Work out the finished part from the listing and answer in its coordinate system (mm). Face numbers are marked on the shaded views. A direction names the side the tool comes from. Round coordinates to 2 decimals unless told otherwise and drop trailing zeros.
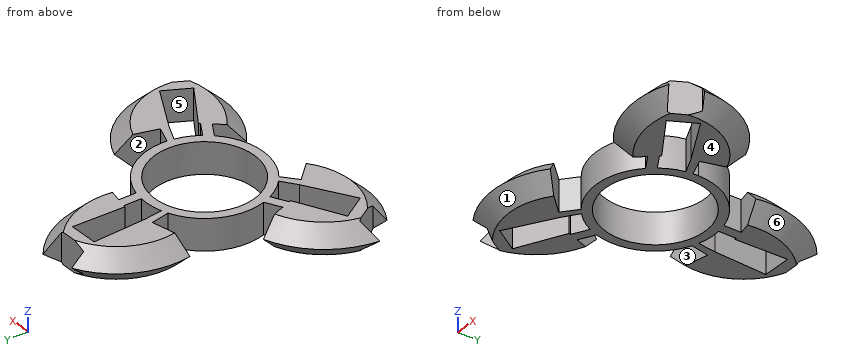
```python
from build123d import *

# Parameters (mm, degrees)
F0_R     = 11.2
F1_DEPTH = 7
F2_SIZE  = 3.5
F3_SIZE  = 3.49999


# Not quite as in the source:
# - a fillet or chamfer is up to 0.001 mm smaller than in the source, because OpenCascade refuses the exact size


with BuildPart() as f1:
    # F0 (on Top) → F1 (new body)
    with BuildSketch(Plane.XY):
        Polygon((-5.4887417888, 30.3404310419), (-5.3626246511, 27.9541106613), (0.7814850479, 28.2788271306), (0.8367048606, 30.6747311771), align=None)
        with BuildLine():
            Line((-6.3603435788, 15.9527909689), (-4.7504720739, 16.3712901342))
            Line((-4.7504720739, 16.3712901342), (-5.3626246511, 27.9541106613))
            Line((-5.3626246511, 27.9541106613), (-5.4887417888, 30.3404310419))
            Line((-5.4887417888, 30.3404310419), (-5.6316571191, 33.0445977541))
            ThreePointArc((-5.6316571191, 33.0445977541), (-13.3586462682, 24.898567552), (-14.7876461409, 13.7620452616))
            Line((-14.7876461409, 13.7620452616), (-6.3603435788, 15.9527909689))
        make_face()
        with BuildLine():
            ThreePointArc((-5.5532608378, 11.975027936), (-4.9107856444, 12.2525174701), (-4.2545066222, 12.4955661497))
            Line((-4.2545066222, 12.4955661497), (-4.7504720739, 16.3712901342))
            Line((-4.7504720739, 16.3712901342), (-6.3603435788, 15.9527909689))
            Line((-6.3603435788, 15.9527909689), (-5.5532608378, 11.975027936))
        make_face()
        with BuildLine():
            Line((0.912733085, 16.988074322), (2.9751978168, 16.625185455))
            Line((2.9751978168, 16.625185455), (8.9877722785, 15.5672782332))
            ThreePointArc((8.9877722785, 15.5672782332), (7.6544413443, 26.2358342161), (0.9277061572, 34.6231396156))
            Line((0.9277061572, 34.6231396156), (0.8367048606, 30.6747311771))
            Line((0.8367048606, 30.6747311771), (0.7814850479, 28.2788271306))
            Line((0.7814850479, 28.2788271306), (0.5228415025, 17.0566754052))
            Line((0.5228415025, 17.0566754052), (0.912733085, 16.988074322))
        make_face()
        with BuildLine():
            ThreePointArc((0.912733085, 13.1684060659), (1.9500586477, 13.055162629), (2.9751978168, 12.8603342861))
            Line((2.9751978168, 12.8603342861), (2.9751978168, 16.625185455))
            Line((2.9751978168, 16.625185455), (0.912733085, 16.988074322))
            Line((0.912733085, 16.988074322), (0.912733085, 13.1684060659))
        make_face()
        with BuildLine():
            ThreePointArc((13.1473088225, -1.1782490086), (13.1868206262, -0.5897132961), (13.2, 0))
            ThreePointArc((13.2, 0), (10.3322943043, 8.214845976), (2.9751978168, 12.8603342861))
            ThreePointArc((2.9751978168, 12.8603342861), (1.9500586477, 13.055162629), (0.912733085, 13.1684060659))
            ThreePointArc((0.912733085, 13.1684060659), (-1.7044180771, 13.089498043), (-4.2545066222, 12.4955661497))
            ThreePointArc((-4.2545066222, 12.4955661497), (-4.9107856444, 12.2525174701), (-5.5532608378, 11.975027936))
            ThreePointArc((-5.5532608378, 11.975027936), (-12.0518959346, 5.3844038094), (-12.6249751013, -3.8535702524))
            ThreePointArc((-12.6249751013, -3.8535702524), (-12.2811318111, -4.8387809867), (-11.8605407229, -5.7937529945))
            ThreePointArc((-11.8605407229, -5.7937529945), (-10.4836287895, -8.020818375), (-8.6942244092, -9.9322938902))
            ThreePointArc((-8.6942244092, -9.9322938902), (-8.1555985672, -10.3791238557), (-7.5940479846, -10.7967789274))
            ThreePointArc((-7.5940479846, -10.7967789274), (1.3629174841, -13.1294499478), (9.6497772845, -9.0067640337))
            ThreePointArc((9.6497772845, -9.0067640337), (10.3310731634, -8.2163816423), (10.9478076379, -7.3746530714))
            ThreePointArc((10.9478076379, -7.3746530714), (12.1880468666, -5.068679668), (12.9487310314, -2.5632722595))
            ThreePointArc((12.9487310314, -2.5632722595), (13.0663842116, -1.8733936144), (13.1473088225, -1.1782490086))
        make_face()
        Circle(F0_R, mode=Mode.SUBTRACT)
        with BuildLine():
            Line((-15.1684704667, -7.7035871225), (-15.885431855, -5.7359958369))
            Line((-15.885431855, -5.7359958369), (-17.975544557, 0))
            ThreePointArc((-17.975544557, 0), (-26.5481195928, -6.4889764521), (-30.4483715445, -16.5081527084))
            Line((-30.4483715445, -16.5081527084), (-26.983448884, -14.6127579238))
            Line((-26.983448884, -14.6127579238), (-24.8809252083, -13.4626276612))
            Line((-24.8809252083, -13.4626276612), (-15.0329349563, -8.0755436793))
            Line((-15.0329349563, -8.0755436793), (-15.1684704667, -7.7035871225))
        make_face()
        with BuildLine():
            ThreePointArc((-11.8605407229, -5.7937529945), (-12.2811318111, -4.8387809867), (-12.6249751013, -3.8535702524))
            Line((-12.6249751013, -3.8535702524), (-15.885431855, -5.7359958369))
            Line((-15.885431855, -5.7359958369), (-15.1684704667, -7.7035871225))
            Line((-15.1684704667, -7.7035871225), (-11.8605407229, -5.7937529945))
        make_face()
        with BuildLine():
            Line((-10.6353504509, -13.4846146005), (-7.5940479846, -10.7967789274))
            ThreePointArc((-7.5940479846, -10.7967789274), (-8.1555985672, -10.3791238557), (-8.6942244092, -9.9322938902))
            Line((-8.6942244092, -9.9322938902), (-11.802717112, -12.2996745631))
            Line((-11.802717112, -12.2996745631), (-10.6353504509, -13.4846146005))
        make_face()
        with BuildLine():
            Line((-4.5244577341, -19.687499851), (-10.6353504509, -13.4846146005))
            Line((-10.6353504509, -13.4846146005), (-11.802717112, -12.2996745631))
            Line((-11.802717112, -12.2996745631), (-21.5276576473, -18.6212245095))
            Line((-21.5276576473, -18.6212245095), (-23.5312131497, -19.9236053449))
            Line((-23.5312131497, -19.9236053449), (-25.8016325533, -21.3994570076))
            ThreePointArc((-25.8016325533, -21.3994570076), (-14.8834688838, -24.0182108044), (-4.5244577341, -19.687499851))
        make_face()
        Polygon((-23.5312131497, -19.9236053449), (-21.5276576473, -18.6212245095), (-24.8809252083, -13.4626276612), (-26.983448884, -14.6127579238), align=None)
        with BuildLine():
            Line((14.2557373817, -9.2844871995), (10.9478076379, -7.3746530714))
            ThreePointArc((10.9478076379, -7.3746530714), (10.3310731634, -8.2163816423), (9.6497772845, -9.0067640337))
            Line((9.6497772845, -9.0067640337), (12.9102340382, -10.8891896181))
            Line((12.9102340382, -10.8891896181), (14.2557373817, -9.2844871995))
        make_face()
        with BuildLine():
            Line((14.5100934538, -8.9811317259), (14.2557373817, -9.2844871995))
            Line((14.2557373817, -9.2844871995), (12.9102340382, -10.8891896181))
            Line((12.9102340382, -10.8891896181), (8.9877722785, -15.5672782332))
            ThreePointArc((8.9877722785, -15.5672782332), (18.8936782485, -19.746857764), (29.5206653873, -18.1149869072))
            Line((29.5206653873, -18.1149869072), (26.1467440233, -16.0619732533))
            Line((26.1467440233, -16.0619732533), (24.0994401604, -14.8161994695))
            Line((24.0994401604, -14.8161994695), (14.5100934538, -8.9811317259))
        make_face()
        Polygon((29.0199549385, -10.416825697), (26.8902822984, -9.3328861518), (24.0994401604, -14.8161994695), (26.1467440233, -16.0619732533), align=None)
        with BuildLine():
            Line((19.312103875, 5.9254545894), (16.9956940297, -2.4681763684))
            Line((16.9956940297, -2.4681763684), (16.5531891859, -4.0716155711))
            Line((16.5531891859, -4.0716155711), (26.8902822984, -9.3328861518))
            Line((26.8902822984, -9.3328861518), (29.0199549385, -10.416825697))
            Line((29.0199549385, -10.416825697), (31.4332896725, -11.6451407465))
            ThreePointArc((31.4332896725, -11.6451407465), (28.242115152, -0.8803567476), (19.312103875, 5.9254545894))
        make_face()
        with BuildLine():
            Line((16.9956940297, -2.4681763684), (13.1473088225, -1.1782490086))
            ThreePointArc((13.1473088225, -1.1782490086), (13.0663842116, -1.8733936144), (12.9487310314, -2.5632722595))
            Line((12.9487310314, -2.5632722595), (16.5531891859, -4.0716155711))
            Line((16.5531891859, -4.0716155711), (16.9956940297, -2.4681763684))
        make_face()
    extrude(amount=F1_DEPTH)

    # F2
    f2_edges = [f1.edges().sort_by_distance(p)[0] for p in [
        (-13.358646, 24.898568, 7),
        (7.654441, 26.235834, 7),
        (28.242115, -0.880357, 7),
        (18.893678, -19.746858, 7),
        (-14.883469, -24.018211, 7),
        (-26.54812, -6.488976, 7),
    ]]
    chamfer(f2_edges, length=F2_SIZE)

    # F3 (size 3.5 in the source; OpenCascade refuses exactly that, so slightly less here)
    f3_edges = [f1.edges().sort_by_distance(p)[0] for p in [
        (7.654441, 26.235834, 0),
        (-13.358646, 24.898568, 0),
        (-26.54812, -6.488976, 0),
        (-14.883469, -24.018211, 0),
        (18.893678, -19.746858, 0),
        (28.242115, -0.880357, 0),
    ]]
    chamfer(f3_edges, length=F3_SIZE)


solid = f1.part
```
1. Which of the six approach directions +Z, -Z, +X, -X, +Y, -Y give full straight-line access (tool end or side, diameter ignored) to the marked faces 1, 2 and 3?
Answer key:
face 1: -Z, -Y
face 2: +Z, -Z, +Y
face 3: +Z, -Z
2. Determine the mould class of the marked faces 4, 5 and 6 for opening direction X: +X half, -X half, draft (parallel to the pull), parting line (faces both ways), or undercut.
Answer key:
face 4: draft
face 5: undercut
face 6: +X half
3. Consider probe 1 along Y at (x, z) = (0, 3.5); probe 2 along Y at (x, z) = (5, 1.5); probe 3 along X at (y, z) = (-4, 1.5). Determine where each line is inside the solid, lowest interval first.
Answer key:
probe 1: y = -13.2 to -11.2, 11.2 to 13.2, 28.24 to 30.63
probe 2: y = -12.22 to -10.02, 10.02 to 12.22, 16.27 to 27.13
probe 3: x = -21.17 to -16.52, -12.88 to -10.46, 10.46 to 12.58, 16.38 to 27.76
4. Given pin 1 (3 mm diameter, centred on y = 14.5, z = 5, fed in from +X); pin 2 (4 mm diameter, centred on y = 18.5, z = 4, fed in from +X); pin 3 (3 mm diameter, centred on x = -7.5, z = 3.5, fed in from +Y), each flat-ended and moving along its own axis, determine where each tip first touches the part or whether it passes through.
Answer key:
pin 1: stops at x = 8.44
pin 2: stops at x = 9.21
pin 3: stops at y = 32.84
